Input: part model. Units: mm. Frame: model coordinates. A direction names the side the tool comes from. Round coordinates to 2 decimals unless told otherwise and drop trailing zeros. Order: outer loops, then holes, each group sorted by start corner. A loop starts at its lowest first (then second) coordinate and runs counter-clockwise, first axis right, second up.
Item 1: Cut plane A-A on x = 0. Output: boundary loops of the cut face in (y, z).
Item 2: Reachability of faces 4 (the cylindrical face through (-8.618, 5.423, 20.784)), 5 (the cylindrical face through (-14.343, 6.916, 25.605)) from +Z, -Z, +X, -X, +Y, -Y: full face, straight path, thin tool, end or side. Return the list, or none.
Item 3: Mould query, pull axis X, two halves, no side actions, for faces 1 (the flat face through (-20, 0, 20)), 2 (the cylindrical face through (23.661, 6.916, 25.605)), 3 (the cylindrical face through (-92.74, 5.42, -20.59)). Classes: released by +X, released by -X, zero draft, split by the parting line, or undercut.
Item 4: Cut plane D-D on z = -37. Output: boundary loops of the cut face in (x, y).
Item 5: Line query: L1, parallel to X at y = 5.25, z = 0; L2, parallel to X at y = 7.75, z = -4.5; L3, parallel to Z at x = 15.5, y = 5. Output: solid intervals per line, ascending.
Item 6: First-contact query: pin 1 (6 mm diameter, centred on x = 35.5, y = 8, fed in from -Z); pin 2 (4 mm diameter, centred on x = 73.5, y = 1.5, fed in from +Z); pin 3 (4 mm diameter, centred on x = -58, y = 9, fed in from -Z). Flat tips, straight axial feed; report the tip coordinate or a pass-through.
Item 7: Cut plane B-B on z = 0. Output: boundary loops of the cut face in (x, y).
Item 8: Cut plane C-C on x = -32. Output: boundary loops of the cut face in (y, z), then the cut area to 3 significant figures.
```python
from build123d import *

# Parameters (mm, degrees)
SKETCH1_R             = 95
BOSS_EXTRUDE1_DEPTH   = 11
SKETCH2_R             = 22.5
CUT_EXTRUDE1_DEPTH    = 135.799851632
SKETCH3_R             = 8.666088256
CUT_EXTRUDE2_DEPTH    = 8.054692
CIRPATTERN1_START     = 2.945308324
CIRPATTERN1_OUTLINE_R = 8.666088256
CIRPATTERN1_DEPTH     = 8.054691676


# Read off the part's stored shape, not the designer's step: CirPattern1
with BuildPart() as part:
    # Sketch1 → Boss-Extrude1 (new body)
    with BuildSketch(Plane(origin=(0, 0, 0), x_dir=(1, 0, 0), z_dir=(0, 1, 0))):
        with Locations(Location((0, 0, 0), (0, 0, 270))):
            Circle(SKETCH1_R)
    extrude(amount=BOSS_EXTRUDE1_DEPTH)

    # Sketch2 → Cut-Extrude1 (cut, through all)
    with BuildSketch(Plane(origin=(0, 0, 0), x_dir=(1, 0, 0), z_dir=(0, 1, 0))):
        with Locations(Location((0, 0, 0), (0, 0, 270))):
            Circle(SKETCH2_R)
    extrude(amount=CUT_EXTRUDE1_DEPTH, mode=Mode.SUBTRACT)

    # Sketch3 → Cut-Extrude2 (cut)
    with BuildSketch(Plane(origin=(0, 11, 0), x_dir=(1, 0, 0), z_dir=(0, 1, 0))):
        with Locations(Location((-38.00433364, 0, 0), (0, 0, 270))):
            Circle(SKETCH3_R)
    extrude(amount=-CUT_EXTRUDE2_DEPTH, mode=Mode.SUBTRACT)

    # CirPattern1 outline → CirPattern1 (cut)
    with BuildSketch(Plane(origin=(0, 0, 0), x_dir=(1, 0, 0), z_dir=(0, 1, 0)).offset(CIRPATTERN1_START)):
        with Locations((-19.00216682, -32.912718386)):
            Circle(CIRPATTERN1_OUTLINE_R)
        with Locations((19.00216682, -32.912718386)):
            Circle(CIRPATTERN1_OUTLINE_R)
        with Locations((38.00433364, 0)):
            Circle(CIRPATTERN1_OUTLINE_R)
        with Locations((19.00216682, 32.912718386)):
            Circle(CIRPATTERN1_OUTLINE_R)
        with Locations((-19.00216682, 32.912718386)):
            Circle(CIRPATTERN1_OUTLINE_R)
    extrude(amount=CIRPATTERN1_DEPTH, mode=Mode.SUBTRACT)


solid = part.part
```
From the geometry:
1. outline: (0, -95) - (11, -95) - (11, -22.5) - (0, -22.5) - close; (0, 22.5) - (11, 22.5) - (11, 95) - (0, 95) - close
2. face 4: +Y, -Y
2. face 5: +Y
3. face 1: zero draft
3. face 2: undercut
3. face 3: split by the parting line
4. outline: (-87.5, 0) - (87.5, 0) - (87.5, 11) - (26.64, 11) - (26.64, 2.95) - (11.36, 2.95) - (11.36, 11) - (-11.36, 11) - (-11.36, 2.95) - (-26.64, 2.95) - (-26.64, 11) - (-87.5, 11) - close
5. L1: x = -95 to -46.67, -29.34 to -22.5, 22.5 to 29.34, 46.67 to 95
5. L2: x = -94.89 to -45.41, -30.6 to -22.05, 22.05 to 30.6, 45.41 to 94.89
5. L3: z = -93.73 to -40.84, -24.99 to -16.31, 16.31 to 24.99, 40.84 to 93.73
6. pin 1: stops at z = -89.27
6. pin 2: stops at z = 62.55
6. pin 3: stops at z = -76.74
7. outline: (-95, 0) - (-22.5, 0) - (-22.5, 11) - (-29.34, 11) - (-29.34, 2.95) - (-46.67, 2.95) - (-46.67, 11) - (-95, 11) - close; (22.5, 0) - (95, 0) - (95, 11) - (46.67, 11) - (46.67, 2.95) - (29.34, 2.95) - (29.34, 11) - (22.5, 11) - close
8. outline: (0, -89.45) - (11, -89.45) - (11, -6.25) - (2.95, -6.25) - (2.95, 6.25) - (11, 6.25) - (11, 89.45) - (0, 89.45) - close
8. area: 1,870 mm2
